Design review of the part built by this model. Coordinates are the model's own, in mm. Coordinates: 2 decimals unless noted, no trailing zeros. Write each loop counter-clockwise with the first axis right and the second up, starting at its lowest first coordinate (ties: lowest second). Pieces come first, ordered by that corner, then holes.
Q1. The part is to be moulded in two halves that separate along Y. For faces 1 (the cylindrical face through (-11.25, 0.07, -0.01)), 2 (the cylindrical face through (-7.43, 7.674, -0.014)), 3 (the flat face through (0, 0, -1)), say which applies: released by +Y, released by -Y, zero draft, split by the parting line, or undercut.
Q2. Take a section at B-B, the plane y = -2.5. Write out the cut boundary in (x, z).
Q3. For L1, parallel to Y at x = 4, z = 0.2 (3 decimals); L2, parallel to X at y = -3.25, z = 0.25; L3, parallel to X at y = -0.5, z = -0.1, list the stretches that pass through material, from the lowest coordinate up.
Q4. Take a section at A-A, the plane x = -4.65. Write out the cut boundary in (y, z) (3 decimals).
Q5. Take a section at C-C, the plane y = 0. Write out the cut boundary in (x, z), plus the area to 3 significant figures.
Q6. Take a section at D-D, the plane x = 3.75. Write out the cut boundary in (y, z) (3 decimals).
Q7. For pin 1 Ø1.8 at (x, y) = (-9.75, 0) entering from +Z; pin 2 Ø0.8 at (y, z) = (-1, 0.5) entering from -X, all flat-tipped, find the tip position at first contact; note any pin that passes through.
from build123d import *

# Parameters (mm, degrees)
SKETCH1_W               = 16
SKETCH1_H               = 16.55
BOSS_EXTRUDE1_DEPTH     = 1
SKETCH2_R               = 1.5
BOSS_EXTRUDE2_DEPTH     = 1
SKETCH3_R               = 1.5
SKETCH3_W               = 3
SKETCH3_H               = 11.5
CUT_EXTRUDE1_DEPTH      = 2
CUT_EXTRUDE1_DEPTH_BACK = 2
FILLET1_R               = 2


with BuildPart() as part:
    # Sketch1 → Boss-Extrude1 (new body, symmetric)
    with BuildSketch(Plane.XY):
        Rectangle(SKETCH1_W, SKETCH1_H)
    extrude(amount=BOSS_EXTRUDE1_DEPTH, both=True)

    # Sketch2 → Boss-Extrude2 (add, symmetric)
    with BuildSketch(Plane.XY):
        with BuildLine():
            Line((-9.75, 4), (-8, 4))
            Line((-8, 4), (-8, -4))
            Line((-8, -4), (-9.75, -4))
            ThreePointArc((-9.75, -4), (-13.75, 0), (-9.75, 4))
        make_face()
        with Locations((-9.75, 0)):
            Circle(SKETCH2_R, mode=Mode.SUBTRACT)
        with BuildLine():
            Line((9.75, -4), (8, -4))
            Line((8, -4), (8, 4))
            Line((8, 4), (9.75, 4))
            ThreePointArc((9.75, 4), (13.75, 0), (9.75, -4))
        make_face()
        with Locations((9.75, 0)):
            Circle(SKETCH2_R, mode=Mode.SUBTRACT)
    extrude(amount=BOSS_EXTRUDE2_DEPTH, both=True)

    # Sketch3 → Cut-Extrude1 (cut, two sides)
    with BuildSketch(Plane.XY) as cut_extrude1_sk:
        with Locations((-4.65, -2.5)):
            Circle(SKETCH3_R)
        with Locations((4.65, 0)):
            Rectangle(SKETCH3_W, SKETCH3_H)
    extrude(amount=CUT_EXTRUDE1_DEPTH, mode=Mode.SUBTRACT)
    extrude(cut_extrude1_sk.sketch, amount=-CUT_EXTRUDE1_DEPTH_BACK, mode=Mode.SUBTRACT)

    # Fillet1
    fillet1_edges = [part.edges().sort_by_distance(p)[0] for p in [
        (-8, -8.275, 0),
        (-8, -4, 0),
        (8, -8.275, 0),
        (8, -4, 0),
        (8, 4, 0),
        (8, 8.275, 0),
        (-8, 8.275, 0),
        (-8, 4, 0),
    ]]
    fillet(fillet1_edges, radius=FILLET1_R)


solid = part.part
Responses:
1. face 1: undercut
1. face 2: released by +Y
1. face 3: zero draft
2. outline: (-12.87, -1) - (-6.15, -1) - (-6.15, 1) - (-12.87, 1) - close; (-3.15, -1) - (3.15, -1) - (3.15, 1) - (-3.15, 1) - close; (6.15, -1) - (12.87, -1) - (12.87, 1) - (6.15, 1) - close
3. L1: y = -8.275 to -5.75, 5.75 to 8.275
3. L2: x = -12.08 to -5.95, -3.35 to 3.15, 6.15 to 12.08
3. L3: x = -13.72 to -11.16, -8.34 to 3.15, 6.15 to 8.34, 11.16 to 13.72
4. outline: (-8.275, -1) - (-4, -1) - (-4, 1) - (-8.275, 1) - close; (-1, -1) - (8.275, -1) - (8.275, 1) - (-1, 1) - close
5. outline: (-13.75, -1) - (-11.25, -1) - (-11.25, 1) - (-13.75, 1) - close; (-8.25, -1) - (3.15, -1) - (3.15, 1) - (-8.25, 1) - close; (6.15, -1) - (8.25, -1) - (8.25, 1) - (6.15, 1) - close; (11.25, -1) - (13.75, -1) - (13.75, 1) - (11.25, 1) - close
5. area: 37.0 mm2
6. outline: (-8.275, -1) - (-5.75, -1) - (-5.75, 1) - (-8.275, 1) - close; (5.75, -1) - (8.275, -1) - (8.275, 1) - (5.75, 1) - close
7. pin 1: passes through
7. pin 2: stops at x = -13.7
